```python
from build123d import *

# Parameters (mm, degrees)
SKETCH1_R           = 1.6
SKETCH1_R_2         = 1.5
BOSS_EXTRUDE1_DEPTH = 3.5
SKETCH2_R           = 7.5
CUT_EXTRUDE1_DEPTH  = 10
BOSS_EXTRUDE2_DEPTH = 6
CUT_EXTRUDE2_DEPTH  = 6
SKETCH5_R           = 1.5
BOSS_EXTRUDE3_DEPTH = 3.5
FILLET1_R           = 3


with BuildPart() as part:
    # Sketch1 → Boss-Extrude1 (new body)
    with BuildSketch(Plane.XY):
        with BuildLine():
            Line((50, -45), (-50, -45))
            ThreePointArc((-50, -45), (-53.535533906, -43.535533906), (-55, -40))
            Line((-55, -40), (-55, 40))
            ThreePointArc((-55, 40), (-53.535533906, 43.535533906), (-50, 45))
            Line((-50, 45), (50, 45))
            ThreePointArc((50, 45), (53.535533906, 43.535533906), (55, 40))
            Line((55, 40), (55, -40))
            ThreePointArc((55, -40), (53.535533906, -43.535533906), (50, -45))
        make_face()
        with Locations((-46.5, 36.5)):
            Circle(SKETCH1_R, mode=Mode.SUBTRACT)
        with Locations((46.5, 36.5)):
            Circle(SKETCH1_R, mode=Mode.SUBTRACT)
        with Locations(Location((46.5, -36.5, 0), (0, 0, 180))):
            Circle(SKETCH1_R, mode=Mode.SUBTRACT)
        with Locations(Location((-46.5, -36.5, 0), (0, 0, 180))):
            Circle(SKETCH1_R, mode=Mode.SUBTRACT)
        with Locations((38.05, 13.55)):
            Circle(SKETCH1_R_2, mode=Mode.SUBTRACT)
        with Locations((38.05, -13.55)):
            Circle(SKETCH1_R_2, mode=Mode.SUBTRACT)
        with Locations(Location((-38.05, -13.55, 0), (0, 0, 180))):
            Circle(SKETCH1_R_2, mode=Mode.SUBTRACT)
        with Locations(Location((-38.05, 13.55, 0), (0, 0, 180))):
            Circle(SKETCH1_R_2, mode=Mode.SUBTRACT)
    extrude(amount=BOSS_EXTRUDE1_DEPTH)

    # Sketch2 → Cut-Extrude1 (cut)
    with BuildSketch(Plane(origin=(0, 0, 0), x_dir=(-1, 0, 0), z_dir=(0, 0, -1))):
        with Locations((0, 30)):
            Circle(SKETCH2_R)
        with BuildLine():
            Line((-15, -15), (15, -15))
            ThreePointArc((15, -15), (18.535533906, -13.535533906), (20, -10))
            Line((20, -10), (20, 10))
            ThreePointArc((20, 10), (18.535533906, 13.535533906), (15, 15))
            Line((15, 15), (-15, 15))
            ThreePointArc((-15, 15), (-18.535533906, 13.535533906), (-20, 10))
            Line((-20, 10), (-20, -10))
            ThreePointArc((-20, -10), (-18.535533906, -13.535533906), (-15, -15))
        make_face()
        with BuildLine():
            Line((1.732050808, -39), (8.660254038, -27))
            ThreePointArc((8.660254038, -27), (8.660254038, -25), (6.92820323, -24))
            Line((6.92820323, -24), (-6.92820323, -24))
            ThreePointArc((-6.92820323, -24), (-8.660254038, -25), (-8.660254038, -27))
            Line((-8.660254038, -27), (-1.732050808, -39))
            ThreePointArc((-1.732050808, -39), (0, -40), (1.732050808, -39))
        make_face()
    extrude(amount=-CUT_EXTRUDE1_DEPTH, mode=Mode.SUBTRACT)

    # Sketch3 → Boss-Extrude2 (add)
    with BuildSketch(Plane.XY.offset(3.5)):
        with BuildLine():
            Line((50, -45), (-50, -45))
            ThreePointArc((-50, -45), (-53.535533906, -43.535533906), (-55, -40))
            Line((-55, -40), (-55, 40))
            ThreePointArc((-55, 40), (-53.535533906, 43.535533906), (-50, 45))
            Line((-50, 45), (50, 45))
            ThreePointArc((50, 45), (53.535533906, 43.535533906), (55, 40))
            Line((55, 40), (55, -40))
            ThreePointArc((55, -40), (53.535533906, -43.535533906), (50, -45))
        make_face()
    extrude(amount=BOSS_EXTRUDE2_DEPTH)

    # Sketch4 → Cut-Extrude2 (cut)
    with BuildSketch(Plane.XY.offset(9.5)):
        with BuildLine():
            Line((47.5, -42.5), (-47.5, -42.5))
            ThreePointArc((-47.5, -42.5), (-51.035533906, -41.035533906), (-52.5, -37.5))
            Line((-52.5, -37.5), (-52.5, 37.5))
            ThreePointArc((-52.5, 37.5), (-51.035533906, 41.035533906), (-47.5, 42.5))
            Line((-47.5, 42.5), (47.5, 42.5))
            ThreePointArc((47.5, 42.5), (51.035533906, 41.035533906), (52.5, 37.5))
            Line((52.5, 37.5), (52.5, -37.5))
            ThreePointArc((52.5, -37.5), (51.035533906, -41.035533906), (47.5, -42.5))
        make_face()
    extrude(amount=-CUT_EXTRUDE2_DEPTH, mode=Mode.SUBTRACT)

    # Sketch5 → Boss-Extrude3 (add)
    # profile 1 of 2: a face of its own
    with BuildSketch(Plane(origin=(0, 0, 0), x_dir=(-1, 0, 0), z_dir=(0, 0, -1))):
        with BuildLine():
            Line((-55, 20), (-64, 20))
            ThreePointArc((-64, 20), (-66.121320344, 19.121320344), (-67, 17))
            Line((-67, 17), (-67, -17))
            ThreePointArc((-67, -17), (-66.121320344, -19.121320344), (-64, -20))
            Line((-64, -20), (-55, -20))
            Line((-55, -20), (-55, 20))
        make_face()
        with Locations((-63.15, 13.55)):
            Circle(SKETCH5_R, mode=Mode.SUBTRACT)
        with Locations((-63.15, -13.55)):
            Circle(SKETCH5_R, mode=Mode.SUBTRACT)
    # profile 2 of 2: a face of its own
    with BuildSketch(Plane(origin=(0, 0, 0), x_dir=(-1, 0, 0), z_dir=(0, 0, -1))):
        with BuildLine():
            Line((64, -20), (55, -20))
            Line((55, -20), (55, 20))
            Line((55, 20), (64, 20))
            ThreePointArc((64, 20), (66.121320344, 19.121320344), (67, 17))
            Line((67, 17), (67, -17))
            ThreePointArc((67, -17), (66.121320344, -19.121320344), (64, -20))
        make_face()
        with Locations(Location((63.15, -13.55, 0), (0, 0, 180))):
            Circle(SKETCH5_R, mode=Mode.SUBTRACT)
        with Locations(Location((63.15, 13.55, 0), (0, 0, 180))):
            Circle(SKETCH5_R, mode=Mode.SUBTRACT)
    extrude(amount=-BOSS_EXTRUDE3_DEPTH)

    # Fillet1
    fillet1_edges = [part.edges().sort_by_distance(p)[0] for p in [
        (55, 20, 1.75),
        (55, -20, 1.75),
        (-55, -20, 1.75),
        (-55, 20, 1.75),
    ]]
    fillet(fillet1_edges, radius=FILLET1_R)


solid = part.part
```
Here's how the part is built. I have some questions about the finished solid (model axes, mm). A direction names the side the tool comes from. Round coordinates to 2 decimals unless told otherwise and drop trailing zeros. Write each loop counter-clockwise with the first axis right and the second up, starting at its lowest first coordinate (ties: lowest second). Pieces come first, ordered by that corner, then holes.
Q1. If we mould it in two halves opening along X, with no side actions, what happens to faces 4 (the cylindrical face through (-66.14, -19.1, 1.73)), 5 (the flat face through (1, 19, 3.5)), 6 (the flat face through (-5.15, -33.08, 1.73)), 7 (the cylindrical face through (54, -43, 5))? For each: +X half, -X half, draft (parallel to the pull), parting line (faces both ways), or undercut.
Q2. If we section it at D-D on y = 13.55: Give the number of separate pieces and of enclosed holes in the cut face, plus the area to 3 significant figures.
Q3. If we section it at C-C on z = 6.75: Write out the boundary of the cut face in (x, y).
Q4. If we section it at B-B on x = 38.05: Write out the boundary of the cut face in (y, z), plus the area to 3 significant figures.
Q5. Please list where these lines run through material, in increasing order: probe 1 along Y at (x, z) = (46.5, 2.8); probe 2 along X at (y, z) = (-37, 4); probe 3 along Y at (x, z) = (-26, 6.75).
Q6. Which directions (+Z, -Z, +X, -X, +Y, -Y) give clear straight access to the entire face, cutting with the end or side of a thin tool? Please do faces 1 (the flat face through (0, 15, 2)), 2 (the cylindrical face through (-51.07, 41, 6.54)), 3 (the cylindrical face through (55.86, -20.9, 1.77)).
Q7. If we section it at A-A on y = -1.5: Write out the boundary of the cut face in (x, z).
Q8. Will these pins go through, and if not, where does the flat tip stop? P1, Ø3.5, axis at x = 38.05, y = 13.55, coming from the +Z side; P2, Ø1.8, axis at y = -18.5, z = 7, coming from the +X side; P3, Ø1.8, axis at x = -61, z = 1.5, coming from the +Y side; P4, Ø2.5, axis at x = -46.5, y = -36.5, coming from the -Z side.
Answer below:
1. face 4: -X half
1. face 5: undercut
1. face 6: undercut
1. face 7: +X half
2. separate pieces: 6
2. enclosed holes: 0
2. area: 327 mm2
3. outline: (-55, -40) arc R5 ccw to (-50, -45) - (50, -45) arc R5 ccw to (55, -40) - (55, 40) arc R5 ccw to (50, 45) - (-50, 45) arc R5 ccw to (-55, 40) - close; hole (-52.5, -37.5) arc R5 ccw to (-47.5, -42.5) - (47.5, -42.5) arc R5 ccw to (52.5, -37.5) - (52.5, 37.5) arc R5 ccw to (47.5, 42.5) - (-47.5, 42.5) arc R5 ccw to (-52.5, 37.5) - close
4. outline: (-45, 0) - (-15.05, 0) - (-15.05, 3.5) - (-42.5, 3.5) - (-42.5, 9.5) - (-45, 9.5) - close; (-12.05, 0) - (12.05, 0) - (12.05, 3.5) - (-12.05, 3.5) - close; (15.05, 0) - (45, 0) - (45, 9.5) - (42.5, 9.5) - (42.5, 3.5) - (15.05, 3.5) - close
4. area: 324 mm2
5. probe 1: y = -45 to -38.1, -34.9 to 34.9, 38.1 to 45
5. probe 2: x = -55 to -52.5, 52.5 to 55
5. probe 3: y = -45 to -42.5, 42.5 to 45
6. face 1: +Z, -Z
6. face 2: +Z
6. face 3: +Z, -Z, +X, -Y
7. outline: (-67, 0) - (-20, 0) - (-20, 3.5) - (-52.5, 3.5) - (-52.5, 9.5) - (-55, 9.5) - (-55, 3.5) - (-67, 3.5) - close; (20, 0) - (67, 0) - (67, 3.5) - (55, 3.5) - (55, 9.5) - (52.5, 9.5) - (52.5, 3.5) - (20, 3.5) - close
8. P1: stops at z = 3.5
8. P2: stops at x = 55
8. P3: stops at y = 20
8. P4: passes through
